Build history of the part. All positions in model axes, mm. A direction names the side the tool comes from. Give positions to 0.01 mm unless a question says otherwise; leave off trailing zeros. Loops run counter-clockwise (first coordinate to the right, second up) from the corner with the lowest first, then second, coordinate; pieces in that order, holes last.
1) Band-saw the part on B-B on z = 0. List the corners of the cut face in (x, y).
2) Wall check: line 1 (X direction, y = 20.6, z = 0); line 2 (Z direction, x = 0, y = 10.25). Give the ranges that are in metal, low to high.
3) Band-saw the part on C-C on y = 2.25. List the corners of the cut face in (x, z), then the cut area to 3 significant figures.
4) Two-plate mould, pull along Z, no slides. Class faces 3 (the flat face through (-1, 21, 1)), 4 (the cylindrical face through (3.233, 10.353, 1.341)), 5 (the cylindrical face through (1.05, 10.35, -0.33)): +Z half, -Z half, draft (parallel to the pull), parting line (faces both ways), or undercut.
5) Band-saw the part on D-D on x = -1.75. List the corners of the cut face in (y, z), then the cut area to 3 significant figures.
6) Flat gauge pins, fed straight in: P1, Ø1, axis at y = 6, z = -2.5, coming from the -X side; P2, Ø2, axis at x = -2, y = 8.5, coming from the -Z side; P3, Ø2, axis at x = -2.5, y = 15, coming from the +Z side. Where does each tip first touch, or does it go through?
7) 3-axis set-ups, long thin cutter, end or side, ignore diameter. For faces 1 (the cylindrical face through (-2.262, 20.014, 1.734)), 2 (the flat face through (1, 0, -1)): which of +Z, -Z, +X, -X, +Y, -Y reach the whole face in a straight line?
8) Band-saw the part on A-A on x = 0. List the corners of the cut face in (y, z), then the cut area to 3 significant figures.
```python
from build123d import *

# Parameters (mm, degrees)
ESQUISSE1_R             = 3.5
ESQUISSE1_R_2           = 1.1
BOSS_EXTRU_2_DEPTH      = 21
ESQUISSE2_R             = 2.85
ESQUISSE2_R_2           = 2.35
ENL_V_MAT_EXTRU_1_DEPTH = 2


with BuildPart() as part:
    # Esquisse1 → Boss.-Extru.2 (new body)
    with BuildSketch(Plane(origin=(0, 0, 0), x_dir=(1, 0, 0), z_dir=(0, 1, 0))):
        Circle(ESQUISSE1_R)
        Circle(ESQUISSE1_R_2, mode=Mode.SUBTRACT)
    extrude(amount=BOSS_EXTRU_2_DEPTH)

    # Esquisse2 → Enlèv. mat.-Extru.1 (cut)
    with BuildSketch(Plane(origin=(0, 21, 0), x_dir=(1, 0, 0), z_dir=(0, 1, 0))):
        Circle(ESQUISSE2_R)
        Circle(ESQUISSE2_R_2, mode=Mode.SUBTRACT)
    extrude(amount=-ENL_V_MAT_EXTRU_1_DEPTH, mode=Mode.SUBTRACT)


solid = part.part
```
Findings below:
1. outline: (-3.5, 0) - (-1.1, 0) - (-1.1, 21) - (-2.35, 21) - (-2.35, 19) - (-2.85, 19) - (-2.85, 21) - (-3.5, 21) - close; (1.1, 0) - (3.5, 0) - (3.5, 21) - (2.85, 21) - (2.85, 19) - (2.35, 19) - (2.35, 21) - (1.1, 21) - close
2. line 1: x = -3.5 to -2.85, -2.35 to -1.1, 1.1 to 2.35, 2.85 to 3.5
2. line 2: z = -3.5 to -1.1, 1.1 to 3.5
3. outline: circle Ø7 at (0, 0); hole circle Ø2.2 at (0, 0)
3. area: 34.7 mm2
4. face 3: draft
4. face 4: parting line
4. face 5: undercut
5. outline: (0, -3.03) - (21, -3.03) - (21, -2.25) - (19, -2.25) - (19, -1.57) - (21, -1.57) - (21, 1.57) - (19, 1.57) - (19, 2.25) - (21, 2.25) - (21, 3.03) - (0, 3.03) - close
5. area: 125 mm2
6. P1: stops at x = -2.87
6. P2: stops at z = -3.35
6. P3: stops at z = 3.16
7. face 1: +Y
7. face 2: +Z, -Z, +X, -X, -Y
8. outline: (0, -3.5) - (21, -3.5) - (21, -2.85) - (19, -2.85) - (19, -2.35) - (21, -2.35) - (21, -1.1) - (0, -1.1) - close; (0, 1.1) - (21, 1.1) - (21, 2.35) - (19, 2.35) - (19, 2.85) - (21, 2.85) - (21, 3.5) - (0, 3.5) - close
8. area: 98.8 mm2
